Input: part model. Units: mm. Frame: model coordinates. A direction names the side the tool comes from. Round coordinates to 2 decimals unless told otherwise and drop trailing zeros. Loops run counter-clockwise (first coordinate to the right, second up) from the corner with the lowest first, then second, coordinate; pieces in that order, holes last. Notation, with made-up numbers: M 59.5,24 L 84.5,24 A31 ccw 84.5,49 Z; hole C -10.5,-14 d11. An arc over 180 degrees is marked long. Use one line per item in the form item = value. Start each with the question number.
Q1. Access query for faces 1 (the cylindrical face through (-10.74, 111.89, -2.38)), 2 (the cylindrical face through (6.64, 226.43, 1.47)). Directions: +Z, -Z, +X, -X, +Y, -Y. A direction counts if a zero-diameter tool reaches every point of the face in a straight line with its end or side. Return the directions, or none.
Q2. Section query A-A, the plane y = 206.5. Output: boundary loops of the cut face in (x, z), and give its area (3 significant figures).
Q3. First-contact query: P1, Ø12, axis at x = 5.5, z = 8, coming from the -Y side; P2, Ø1.1, axis at y = 226.5, z = 0, coming from the -X side; P3, Ø1, axis at x = 8, y = 203.5, coming from the -Z side. Flat tips, straight axial feed; report the tip coordinate or a pass-through.
Q4. Ray query, line 1 along Y through (x, z) = (3.65, 0); line 2 along Z through (x, y) = (0.25, 153); line 3 along Y through (x, z) = (5, 0). Return the intervals inside material, ascending.
```python
from build123d import *

# Parameters (mm, degrees)
SKETCH1_R           = 11
BOSS_EXTRUDE1_DEPTH = 216.66667
BOSS_EXTRUDE2_START = 216.66667
SKETCH2_R           = 6.8
BOSS_EXTRUDE2_DEPTH = 19.8
FILLET1_R           = 10
CUT_EXTRUDE1_START  = -1.44
SKETCH3_R           = 0.5
CUT_EXTRUDE1_DEPTH  = 9
CUT_EXTRUDE2_START  = -1.4
SKETCH4_R           = 0.5
CUT_EXTRUDE2_DEPTH  = 9


with BuildPart() as part:
    # Sketch1 → Boss-Extrude1 (new body)
    with BuildSketch(Plane(origin=(0, 0, 0), x_dir=(1, 0, 0), z_dir=(0, 1, 0))):
        with Locations(Location((0, 0, 0), (0, 0, 270))):
            Circle(SKETCH1_R)
    extrude(amount=BOSS_EXTRUDE1_DEPTH)

    # Sketch2 → Boss-Extrude2 (add)
    with BuildSketch(Plane(origin=(0, 0, 0), x_dir=(1, 0, 0), z_dir=(0, 1, 0)).offset(BOSS_EXTRUDE2_START)):
        with Locations(Location((0, 0, 0), (0, 0, 90))):
            Circle(SKETCH2_R)
    extrude(amount=BOSS_EXTRUDE2_DEPTH)

    # Fillet1
    fillet1_edges = [part.edges().sort_by_distance(p)[0] for p in [
        (0, 0, -11),
    ]]
    fillet(fillet1_edges, radius=FILLET1_R)

    # Sketch3 → Cut-Extrude1 (cut)
    with BuildSketch(Plane.XY.offset(CUT_EXTRUDE1_START)):
        with Locations((0, 231.66667)):
            Circle(SKETCH3_R)
    cut_extrude1 = extrude(amount=-CUT_EXTRUDE1_DEPTH, mode=Mode.SUBTRACT)

    # Mirror1: Cut-Extrude1 across plane
    add(cut_extrude1.mirror(Plane.XY), mode=Mode.SUBTRACT)

    # Sketch4 → Cut-Extrude2 (cut)
    with BuildSketch(Plane(origin=(0, 0, 0), x_dir=(0, 0, -1), z_dir=(1, 0, 0)).offset(CUT_EXTRUDE2_START)):
        with Locations((0, 226.66667)):
            Circle(SKETCH4_R)
    cut_extrude2 = extrude(amount=-CUT_EXTRUDE2_DEPTH, mode=Mode.SUBTRACT)

    # Mirror2: Cut-Extrude2 across plane
    add(cut_extrude2.mirror(Plane(origin=(0, 0, 0), x_dir=(0, 0, 1), z_dir=(1, 0, 0))), mode=Mode.SUBTRACT)


solid = part.part
```
Results found:
q1.face_1 = +Y, -Y
q1.face_2 = +Y
q2.outline = C 0,0 d22
q2.area = 380 mm²
q3.P1 = 0.37
q3.P2 = -6.8
q3.P3 = -8.05
q4.line_1 = 0.36 to 226.17, 227.17 to 236.47
q4.line_2 = -11 to 11
q4.line_3 = 0.83 to 226.17, 227.17 to 236.47
